```python
from build123d import *

# Parameters (mm, degrees)
SKETCH1_W                   = 236
SKETCH1_H                   = 69
SKETCH1_W_2                 = 232
SKETCH1_H_2                 = 65
DISPLAY_OUTLINE_DEPTH       = 5
SKETCH3_W                   = 236
SKETCH3_H                   = 69
SKETCH3_W_2                 = 226
SKETCH3_H_2                 = 59
REAR_DISPLAY_RETAINER_DEPTH = 2
SKETCH2_W                   = 74
SKETCH2_H                   = 111.25
SKETCH2_W_2                 = 70
SKETCH2_H_2                 = 107.25
STREAM_DECK_OUTLINE_DEPTH   = 9
STREAM_DECK_RETAINER_DEPTH  = 2


with BuildPart() as part:
    # Sketch1 → Display outline (new body)
    with BuildSketch(Plane.XY):
        Rectangle(SKETCH1_W, SKETCH1_H)
        Rectangle(SKETCH1_W_2, SKETCH1_H_2, mode=Mode.SUBTRACT)
    extrude(amount=DISPLAY_OUTLINE_DEPTH)

    # Sketch3 → Rear display retainer (add)
    with BuildSketch(Plane(origin=(0, 0, 0), x_dir=(-1, 0, 0), z_dir=(0, 0, -1))):
        Rectangle(SKETCH3_W, SKETCH3_H)
        Rectangle(SKETCH3_W_2, SKETCH3_H_2, mode=Mode.SUBTRACT)
    extrude(amount=REAR_DISPLAY_RETAINER_DEPTH)

    # Sketch2 → Stream deck outline (add)
    with BuildSketch(Plane(origin=(27.334936491, 0, -47.345498823), x_dir=(0, 1, 0), z_dir=(-0.5000000000000041, 0, 0.8660254037844364))):
        with Locations((0.5, -158.315997647)):
            Rectangle(SKETCH2_W, SKETCH2_H)
        with Locations((0.5, -158.315997647)):
            Rectangle(SKETCH2_W_2, SKETCH2_H_2, mode=Mode.SUBTRACT)
    extrude(amount=-STREAM_DECK_OUTLINE_DEPTH)

    # Sketch4 → Stream deck retainer (add)
    with BuildSketch(Plane(origin=(31.834936491, 0, -55.139727457), x_dir=(-0.8660254037844363, 0, -0.5000000000000042), z_dir=(0.5000000000000041, 0, -0.8660254037844362))):
        with BuildLine():
            Line((-213.940997647, 27.5), (-205.940997647, 27.5))
            ThreePointArc((-205.940997647, 27.5), (-204.526784084, 28.085786438), (-203.940997647, 29.5))
            Line((-203.940997647, 29.5), (-203.940997647, 32.5))
            ThreePointArc((-203.940997647, 32.5), (-203.355211209, 33.914213562), (-201.940997647, 34.5))
            Line((-201.940997647, 34.5), (-179.940997647, 34.5))
            ThreePointArc((-179.940997647, 34.5), (-178.526784084, 33.914213562), (-177.940997647, 32.5))
            Line((-177.940997647, 32.5), (-177.940997647, 29.5))
            ThreePointArc((-177.940997647, 29.5), (-177.355211209, 28.085786438), (-175.940997647, 27.5))
            Line((-175.940997647, 27.5), (-102.690997647, 27.5))
            Line((-102.690997647, 27.5), (-102.690997647, 37.5))
            Line((-102.690997647, 37.5), (-213.940997647, 37.5))
            Line((-213.940997647, 37.5), (-213.940997647, 27.5))
        make_face()
        with BuildLine():
            Line((-102.690997647, -36.5), (-102.690997647, -26.5))
            Line((-102.690997647, -26.5), (-183.940997647, -26.5))
            ThreePointArc((-183.940997647, -26.5), (-185.355211209, -27.085786438), (-185.940997647, -28.5))
            Line((-185.940997647, -28.5), (-185.940997647, -31.5))
            ThreePointArc((-185.940997647, -31.5), (-186.526784084, -32.914213562), (-187.940997647, -33.5))
            Line((-187.940997647, -33.5), (-192.940997647, -33.5))
            ThreePointArc((-192.940997647, -33.5), (-194.355211209, -32.914213562), (-194.940997647, -31.5))
            Line((-194.940997647, -31.5), (-194.940997647, -28.5))
            ThreePointArc((-194.940997647, -28.5), (-195.526784084, -27.085786438), (-196.940997647, -26.5))
            Line((-196.940997647, -26.5), (-213.940997647, -26.5))
            Line((-213.940997647, -26.5), (-213.940997647, -36.5))
            Line((-213.940997647, -36.5), (-102.690997647, -36.5))
        make_face()
    extrude(amount=STREAM_DECK_RETAINER_DEPTH)


solid = part.part
```
Verification items for the finished model (mm, model axes). A direction names the side the tool comes from. Round coordinates to 2 decimals unless told otherwise and drop trailing zeros. Order: outer loops, then holes, each group sorted by start corner. A loop starts at its lowest first (then second) coordinate and runs counter-clockwise, first axis right, second up. Notation, with made-up numbers: (9.5, -17) - (35.5, -17) arc R23 ccw to (35.5, 3) - close; hole circle Ø1 at (-8.5, 6). An arc over 180 degrees is marked (long way). Use CSV: the item, a comma, the result in double quotes. Start each with the question number.
1) Thickness scan on L1, parallel to Y at x = -96, z = -1; L2, parallel to X at y = 10, z = -0.5; L3, parallel to X at y = 31, z = 25.5. Record the ranges inside material, lowest first.
2) Go/stop test with flat-tipped pins: P1, Ø2, axis at y = 12, z = -0.5, coming from the +X side; P2, Ø5.5, axis at x = -15, z = 1, coming from the -Y side; P3, Ø4, axis at x = 202.5, z = 36.5, coming from the -Y side; P4, Ø0.9, axis at y = 9.5, z = -1, coming from the +X side. Record where each tip stops, or that it passes through.
3) Access from +Z, -Z, +X, -X, +Y, -Y to the whole of each face (thin tool, end or side, straight path). Record for faces 4 (the flat face through (1, 31, 0)), 5 (the flat face through (213.1, 0.01, 54.78)), 6 (the flat face through (168, -36.5, 28)), 7 (the flat face through (9, -31, -2)).
4) Section check C-C, the plane z = 8.5. Record the cut outline in (x, y), plus the area to 3 significant figures.
5) Mould release check, pull along Y, two halves, no side actions. Record for faces 1 (the flat face through (-118, 0, 2)), 2 (the flat face through (2, -34.5, 2)), 3 (the flat face through (120.219, 0.01, 1.157)): +Y half, -Y half, draft (parallel to the pull), parting line (faces both ways), or undercut.
6) Section check D-D, the plane z = 55.5. Record the cut outline in (x, y).
7) Section check A-A, the plane x = -74. Record the cut outline in (y, z), plus the area to 3 significant figures.
8) Section check B-B, the plane y = 11.5. Record the cut outline in (x, z) (3 decimals), plus the area to 3 significant figures.
Answers:
1,L1,"y = -34.5 to -29.5, 29.5 to 34.5"
1,L2,"x = -118 to -113, 113 to 118, 118.87 to 121.18"
1,L3,"x = 171.51 to 175.51"
2,P1,"stops at x = 121.75"
2,P2,"stops at y = -34.5"
2,P3,"passes through"
2,P4,"stops at x = 121.72"
3,face 4,"+Z"
3,face 5,"-X"
3,face 6,"+Z, -Z, +X, -X, -Y"
3,face 7,"-Z, -X, +Y, -Y"
4,outline,"(124.06, -36.5) - (146.06, -36.5) - (146.06, -26.5) - (142.06, -26.5) - (142.06, -34.5) - (124.06, -34.5) - close; (124.06, 35.5) - (142.06, 35.5) - (142.06, 27.5) - (146.06, 27.5) - (146.06, 37.5) - (124.06, 37.5) - close"
4,area,"152 mm²"
5,face 1,"draft"
5,face 2,"-Y half"
5,face 3,"undercut"
6,outline,"(205.47, -36.5) - (214.99, -36.5) - (214.99, 37.5) - (205.47, 37.5) - (205.47, 35.5) - (212.69, 35.5) - (212.69, -34.5) - (205.47, -34.5) - close"
7,outline,"(-34.5, -2) - (-29.5, -2) - (-29.5, 0) - (-32.5, 0) - (-32.5, 5) - (-34.5, 5) - close; (29.5, -2) - (34.5, -2) - (34.5, 5) - (32.5, 5) - (32.5, 0) - (29.5, 0) - close"
7,area,"40.0 mm²"
8,outline,"(-118, -2) - (-113, -2) - (-113, 0) - (-116, 0) - (-116, 5) - (-118, 5) - close; (113, -2) - (118, -2) - (118, 1) - (120.768, -3.794) - (122.5, -2.794) - (118, 5) - (116, 5) - (116, 0) - (113, 0) - close; (210.881, 58.625) - (215.381, 50.831) - (217.113, 51.831) - (212.613, 59.625) - close"
8,area,"72.5 mm²"
